Verification items for the finished model (mm, model axes). A direction names the side the tool comes from. Round coordinates to 2 decimals unless told otherwise and drop trailing zeros. Write item = value, one per line.
Solid Edge part; units mm, degrees
sketch "Sketch1" plane through (0, 0, 0) normal (1, 0, 0) x (0, 1, 0)
  line L0 (4, 0) -> (4, 37.5)
  line L1 (4, 37.5) -> (-2, 37.5)
  line L2 (-2, 37.5) -> (-4, 35.5)
  line L3 (-4, 35.5) -> (-4, 0)
  dimension "D1" = 4
  dimension "D2" = 4
revolve "RevolvedProtrusion1" add sketch "Sketch1" angle 360 about axis through (0, -4, 0) along (0, 1, 0)
hole "Hole_1" at (30, 4, 10) direction (0, -1, 0) diameter 4 end up to next
hole "Hole1" at (-30, 4, 10) direction (0, -1, 0) diameter 4 end up to next
hole "Hole2" at (0, 4, -30) direction (0, -1, 0) diameter 4 end up to next
hole "Hole_4" at (0, 4, 25) direction (0, -1, 0) diameter 4.8 end up to next counterbore diameter 8 counterbore depth 4.8
hole "Hole3" at (0, 4, -25) direction (0, -1, 0) diameter 4.8 end up to next counterbore diameter 8 counterbore depth 4.8
hole "Hole4" at (-21.6506, 4, 12.5) direction (0, -1, 0) diameter 4.8 end up to next counterbore diameter 8 counterbore depth 4.8
hole "Hole5" at (-21.6506, 4, -12.5) direction (0, -1, 0) diameter 4.8 end up to next counterbore diameter 8 counterbore depth 4.8
hole "Hole6" at (21.6506, 4, 12.5) direction (0, -1, 0) diameter 4.8 end up to next counterbore diameter 8 counterbore depth 4.8
hole "Hole7" at (21.6506, 4, -12.5) direction (0, -1, 0) diameter 4.8 end up to next counterbore diameter 8 counterbore depth 4.8
properties material "Polyethylene, low density"
(1) Go/stop test with flat-tipped pins: pin 1 Ø6.5 at (x, z) = (-22, -12.5) entering from +Y; pin 2 Ø2 at (x, y) = (22.5, 0.5) entering from +Z; pin 3 Ø4.5 at (x, z) = (-30, 10) entering from -Y; pin 4 Ø4 at (x, y) = (-6.5, 0.5) entering from +Z. Record where each tip stops, or that it passes through.
Filled sheet:
pin_1 = -0.8
pin_2 = 30.72
pin_3 = -4
pin_4 = 37.23
(2) Material ranges on probe 1 along Z at (x, y) = (-21, 2.5); probe 2 along X at (y, z) = (0.5, -16); probe 3 along X at (y, z) = (1.75, -14.5), recorded low to high. Write a range as from..to.
Filled sheet:
probe_1 = -31.07..-16.45, -8.55..8.55, 16.45..31.07
probe_2 = -33.92..-23.59, -19.71..19.71, 23.59..33.92
probe_3 = -34.58..-25.11, -18.19..18.19, 25.11..34.58
(3) Sectioned sample at A-A, the plane y = 2.75. Count the separate pieces of the cut face and the enclosed holes in it, and give its area (3 significant figures).
Filled sheet:
separate_pieces = 1
enclosed_holes = 8
area = 4,080 mm2
(4) Set-up check for faces 1 (the face through (2, -0.8, 27)), 2 (the face through (-23.994, -2.378, 11.98)): record each of +Z, -Z, +X, -X, +Y, -Y from which the full face is reachable in a straight line by a thin tool's end or side.
Filled sheet:
face_1 = +Y
face_2 = +Y, -Y
(5) Draft check along X on faces 3 (the face through (2, -0.8, -23)), 4 (the face through (0, -4, 0)), 5 (the face through (-34.778, -3.875, -7.723)). Enter one of: released by +X, released by -X, zero draft, split by the parting line, or undercut.
Filled sheet:
face_3 = undercut
face_4 = zero draft
face_5 = split by the parting line
